Autodesk Inventor part; units mm, degrees
ref_plane "YZ Plane" through (0, 0, 0) normal (1, 0, 0) x (0, 1, 0)
ref_plane "XZ Plane" through (0, 0, 0) normal (0, 1, 0) x (-1, 0, 0)
ref_plane "XY Plane" through (0, 0, 0) normal (0, 0, 1) x (1, 0, 0)
sketch "Sketch1" plane through (0, 0, 0) normal (0, 0, 1) x (1, 0, 0)
  line L0 (0, 0) -> (0, 100)
  line L1 (0, 100) -> (-20, 100)
  line L2 (-20, 100) -> (-20, 60)
  line L3 (-20, 60) -> (-80, 60)
  line L4 (-80, 60) -> (-80, 40)
  line L5 (-80, 40) -> (-20, 40)
  line L6 (-20, 40) -> (-20, 0)
  line L7 (-20, 0) -> (0, 0)
  dimension "d0" = 20
  dimension "d1" = 100
  dimension "d2" = 20
  dimension "d3" = 40
  dimension "d4" = 60
extrude "Extrusion1" add sketch "Sketch1" along normal blind 6
sketch "Sketch2" plane through (0, 0, 6) normal (0, 0, 1) x (1, 0, 0)
  line L0 (0, 100) -> (-20, 100)
  line L1 (-20, 60) -> (-80, 60)
  line L2 (-80, 40) -> (-20, 40)
  line L3 (-20, 0) -> (0, 0)
  line L4 (-20, 40) -> (-20, 0)
  line L5 (-20, 100) -> (-20, 60)
  line L6 (-80, 60) -> (-80, 40)
  point P0 (-10, 93)
  point P1 (-10, 67)
  point P2 (-10, 33)
  point P3 (-10, 7)
  point P4 (-73, 50.2147)
  point P5 (-50, 50.2147)
  point P6 (-27, 50.2147)
  dimension "d7" = 7
  dimension "d8" = 7
  dimension "d9" = 7
  dimension "d10" = 7
  dimension "d11" = 10
  dimension "d12" = 10
  dimension "d13" = 10
  dimension "d14" = 10
  dimension "d15" = 7
  dimension "d16" = 7
  dimension "d17" = 23
hole "Hole1" at (-10, 93, 6) at (-10, 67, 6) at (-10, 33, 6) at (-10, 7, 6) at (-73, 50.2147, 6) at (-50, 50.2147, 6) at (-27, 50.2147, 6) direction (0, 0, -1) diameter 5 depth 8 tip angle 118
properties part number "side corner brackets"
CAD build for the part. Positions are in the model's coordinates, mm. A direction names the side the tool comes from. Give positions to 0.01 mm unless a question says otherwise; leave off trailing zeros. Write each loop counter-clockwise with the first axis right and the second up, starting at its lowest first coordinate (ties: lowest second). Pieces come first, ordered by that corner, then holes. Notation, with made-up numbers: M 87,23 L 132,23 A5 ccw 132,29 Z; hole C 44.5,-12 d7. An arc over 180 degrees is marked long. Return JSON: item names as keys, results as strings. Group by question number.
(1) Band-saw the part on A-A (x = -73). Give the cut face in (y, z).
(2) Mould opens along X. For faces 4 (the face through (-10, 100, 3)), 5 (the face through (-7.78, 5.85, 2.96)), 6 (the face through (0, 49, 3)) say: pulls with the +X half, pulls with the -X half, needs draft (parallel to the pull), parting line crosses it, or undercut.
(3) Band-saw the part on D-D (z = 2.1). Give the cut face in (x, y).
(4) Band-saw the part on C-C (x = -10). Give the cut face in (y, z), and give its area (3 significant figures).
(5) Drill centre lines: L1, parallel to Y at x = -10, z = 3.4; L2, parallel to Y at x = -27, z = 5.75; L3, parallel to X at y = 7, z = 3.8. Where is each one in solid material? Low to high. Write a range as [from, to].
(6) Band-saw the part on B-B (y = 7). Give the cut face in (x, z).
(7) 3-axis set-ups, long thin cutter, end or side, ignore diameter. For faces 1 (the face through (-50, 60, 3)), 2 (the face through (-7.78, 65.85, 2.96)), 3 (the face through (-20, 20, 3)): which of +Z, -Z, +X, -X, +Y, -Y reach the whole face in a straight line?
(8) Flat gauge pins, fed straight in: pin 1 Ø4.5 at (x, y) = (-27, 50.21) entering from +Z; pin 2 Ø1.8 at (y, z) = (22.5, 2.5) entering from -X. Where does each tip first touch, or does it go through?
Entries:
{
 "1": {"outline": "M 40,0 L 47.71,0 L 47.71,6 L 40,6 Z; M 52.71,0 L 60,0 L 60,6 L 52.71,6 Z"},
 "2": {"face 4": "needs draft", "face 5": "undercut", "face 6": "pulls with the +X half"},
 "3": {"outline": "M -80,40 L -20,40 L -20,0 L 0,0 L 0,100 L -20,100 L -20,60 L -80,60 Z; hole C -73,50.21 d5; hole C -50,50.21 d5; hole C -27,50.21 d5; hole C -10,7 d5; hole C -10,33 d5; hole C -10,67 d5; hole C -10,93 d5"},
 "4": {"outline": "M 0,0 L 4.5,0 L 4.5,6 L 0,6 Z; M 9.5,0 L 30.5,0 L 30.5,6 L 9.5,6 Z; M 35.5,0 L 64.5,0 L 64.5,6 L 35.5,6 Z; M 69.5,0 L 90.5,0 L 90.5,6 L 69.5,6 Z; M 95.5,0 L 100,0 L 100,6 L 95.5,6 Z", "area": "480 mm^2"},
 "5": {"L1": "y = [0, 4.5], [9.5, 30.5], [35.5, 64.5], [69.5, 90.5], [95.5, 100]", "L2": "y = [40, 47.71], [52.71, 60]", "L3": "x = [-20, -12.5], [-7.5, 0]"},
 "6": {"outline": "M -20,0 L -12.5,0 L -12.5,6 L -20,6 Z; M -7.5,0 L 0,0 L 0,6 L -7.5,6 Z"},
 "7": {"face 1": "+Z, -Z, -X, +Y", "face 2": "+Z, -Z", "face 3": "+Z, -Z, -X, -Y"},
 "8": {"pin 1": "passes through", "pin 2": "stops at x = -20"}
}
